CAD build for the part. Positions are in the model's coordinates, mm. A direction names the side the tool comes from. Give positions to 0.01 mm unless a question says otherwise; leave off trailing zeros. Write each loop counter-clockwise with the first axis right and the second up, starting at its lowest first coordinate (ties: lowest second). Pieces come first, ordered by that corner, then holes. Notation, with made-up numbers: (-35, 78.25) -> (15, 78.25) arc R29 ccw to (15, 115.25) -> close; hole circle Ø3 at (72, -12). An arc over 180 degrees is marked (long way). Use one line per item in the form item = value. Start each with the question number.
from build123d import *
from OCP.BRepFilletAPI import BRepFilletAPI_MakeChamfer

# Parameters (mm, degrees)
BOSS_EXTRUDE1_DEPTH = 18
BOSS_EXTRUDE2_DEPTH = 50
CHAMFER1_SIZE       = 4
CHAMFER1_SIZE2      = 4.182741942
FILLET1_R           = 10


with BuildPart() as part:
    # Sketch1 → Boss-Extrude1 (new body)
    with BuildSketch(Plane.XY):
        Polygon((0, 0), (68.2, 0), (64, -98.1), (4.2, -98.1), align=None)
    extrude(amount=BOSS_EXTRUDE1_DEPTH)

    # Sketch2 → Boss-Extrude2 (add)
    with BuildSketch(Plane(origin=(0, 0, 0), x_dir=(-1, 0, 0), z_dir=(0, 0, -1))):
        Polygon((-62.16942167, -94.1), (-6.03057833, -94.1), (-3.391390108, -32.456103661), (-64.808609892, -32.456103661), align=None)
    extrude(amount=BOSS_EXTRUDE2_DEPTH)

    # Chamfer1: one chamfer whose edges measure the first distance from different faces: ONE call of the kernel's chamfer builder (chamfer() names one face for all edges)
    chamfer1_edges_1 = [part.edges().sort_by_distance(p)[0] for p in [
        (64, -98.1, 9),
    ]]
    chamfer1_side_1 = [part.faces().sort_by_distance(p)[0] for p in [
        (34.1, -98.1, 9),
    ]]
    chamfer1_edges_2 = [part.edges().sort_by_distance(p)[0] for p in [
        (4.2, -98.1, 9),
    ]]
    chamfer1_side_2 = [part.faces().sort_by_distance(p)[0] for p in [
        (2.1, -49.05, 9),
    ]]
    chamfer1 = BRepFilletAPI_MakeChamfer(part.part.solid().wrapped)
    for e in chamfer1_edges_1:
        chamfer1.Add(CHAMFER1_SIZE, CHAMFER1_SIZE2, e.wrapped, chamfer1_side_1[0].wrapped)  # the first distance lies on this face
    for e in chamfer1_edges_2:
        chamfer1.Add(CHAMFER1_SIZE, CHAMFER1_SIZE2, e.wrapped, chamfer1_side_2[0].wrapped)  # the first distance lies on this face
    add(Compound.cast(chamfer1.Shape()), mode=Mode.REPLACE)

    # Fillet1
    fillet1_edges = [part.edges().sort_by_distance(p)[0] for p in [
        (63.489015781, -63.27805183, -50),
        (34.1, -94.1, -50),
        (4.710984219, -63.27805183, -50),
        (34.1, -32.456103661, -50),
    ]]
    fillet(fillet1_edges, radius=FILLET1_R)


solid = part.part
1) Cut at A-A (x = 34.5). Give the cut face in (y, z), and give its area (3 significant figures).
2) 3-axis set-ups, long thin cutter, end or side, ignore diameter. For faces 1 (the face through (34, -94.1, -20)), 2 (the face through (4.73, -63.71, -19.72)), 3 (the face through (63.507, -62.847, -19.72)): which of +Z, -Z, +X, -X, +Y, -Y reach the whole face in a straight line?
3) Cut at C-C (y = -10). Give the cut face in (x, z).
4) Wall check: line 1 along Y through (x, z) = (42, -1); line 2 along Z through (x, y) = (22.5, -15); line 3 along X through (y, z) = (-33, -31.5). Give the ranges that are in metal, low to high. Write a range as from..to.
5) Cut at B-B (z = -5). Give the cut face in (x, y).
6) Pin check, flat tips, straight feed: pin 1 (4 mm diameter, centred on y = -67.5, z = -18.5, fed in from -X); pin 2 (3 mm diameter, centred on y = -57.5, z = -22.5, fed in from -X); pin 3 (5 mm diameter, centred on x = 22.5, z = 4, fed in from +Y); pin 4 (8 mm diameter, centred on y = -24.5, z = -18, fed in from -X). Stop position of each tip, or through.
Final values:
q1.outline = (-98.1, 0) -> (-94.1, 0) -> (-94.1, -40) arc R10 ccw to (-84.1, -50) -> (-42.46, -50) arc R10 ccw to (-32.46, -40) -> (-32.46, 0) -> (0, 0) -> (0, 18) -> (-98.1, 18) -> close
q1.area = 4,810 mm^2
q2.face_1 = -Z, +X, -X, -Y
q2.face_2 = -Z, -X, -Y
q2.face_3 = -Z, +X, -Y
q3.outline = (0.43, 0) -> (67.77, 0) -> (67.77, 18) -> (0.43, 18) -> close
q4.line_1 = -94.1..-32.46
q4.line_2 = 0..18
q4.line_3 = 3.41..64.79
q5.outline = (3.39, -32.46) -> (6.03, -94.1) -> (62.17, -94.1) -> (64.81, -32.46) -> close
q6.pin_1 = 4.81
q6.pin_2 = 4.4
q6.pin_3 = 0
q6.pin_4 = through
